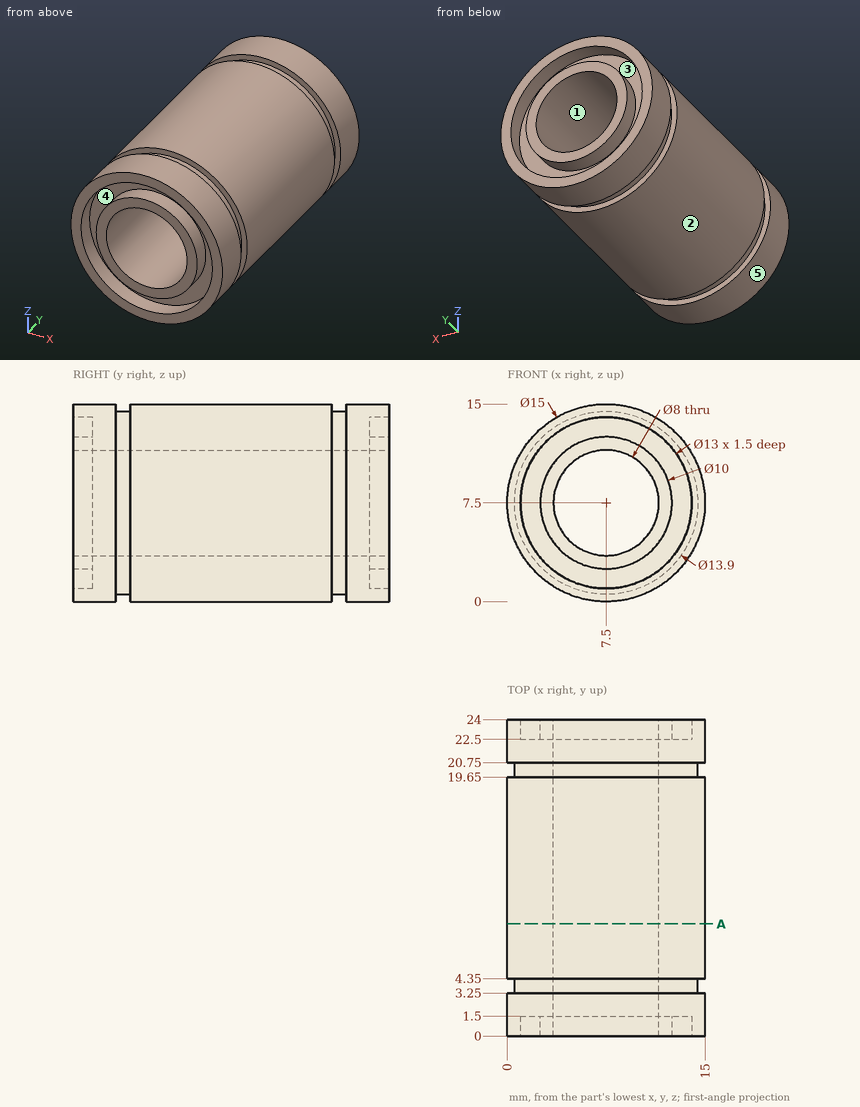
Job drawing, mm, ordinate dimensions from the low corner. One solid piece. A direction names the side the tool comes from. Give positions to 0.01 mm unless a question says otherwise; leave off trailing zeros. Order: outer loops, then holes, each group sorted by start corner. A loop starts at its lowest first (then second) coordinate and runs counter-clockwise, first axis right, second up. Notation, with made-up numbers: M 20.5,-35.5 L 76.5,-35.5 A31 cw 76.5,2.5 Z; hole C 51.5,52.25 d6. An arc over 180 degrees is marked long. Put each result on its own line as item: value. Start each with the question number.
(1) Drill centre lines: L1, parallel to Z at x = 7.5, y = 22.95; L2, parallel to Y at x = 11.5, z = 1.5; L3, parallel to Z at x = 7.5, y = 13.75. Where is each one in solid material? Low to high. Write a range as [from, to].
(2) Pull direction Z, two halves, no side cores. Call the marked faces 1 and 2: released by +Z, released by -Z, zero draft, split by the parting line, or undercut.
(3) Pin check, flat tips, straight feed: pin 1 Ø4 at (x, y) = (10, 13.5) entering from -Z; pin 2 Ø6.5 at (x, z) = (7.5, 7.5) entering from +Y; pin 3 Ø1.5 at (x, y) = (4.5, 6.5) entering from +Z. Stop position of each tip, or through.
(4) Tool access for the marked faces 3, 4 and 5: list every direction of +Z, -Z, +X, -X, +Y, -Y with a clear straight run to the whole face (end or side of a thin tool).
(5) Band-saw the part on A-A on y = 8.5. Give the cut face in (x, z), then the cut area to 3 significant figures.
Results below:
1. L1: z = [0, 1], [2.5, 3.5], [11.5, 12.5], [14, 15]
1. L2: y = [0, 3.25], [4.35, 19.65], [20.75, 24]
1. L3: z = [0, 3.5], [11.5, 15]
2. face 1: undercut
2. face 2: split by the parting line
3. pin 1: stops at z = 0.02
3. pin 2: passes through
3. pin 3: stops at z = 14.65
4. face 3: +Y
4. face 4: -Y
4. face 5: +Y, -Y
5. outline: C 7.5,7.5 d15; hole C 7.5,7.5 d8
5. area: 126 mm2
